Geometry: final body of the model. Coordinates: model frame, mm. Give positions to 0.01 mm unless a question says otherwise; leave off trailing zeros. Write each loop counter-clockwise with the first axis right and the second up, starting at its lowest first coordinate (ties: lowest second). Pieces come first, ordered by that corner, then holes. Notation, with made-up numbers: (26.5, 81.25) - (31.5, 81.25) arc R36 cw to (31.5, 116.25) - close; hole circle Ø6 at (76, 65). An arc over 180 degrees is marked (long way). Return JSON: item names as keys, results as strings.
from build123d import *

# Parameters (mm, degrees)
SKETCH1_R           = 2.5
BOSS_EXTRUDE1_DEPTH = 6.2
SKETCH2_R           = 2.5
CUT_EXTRUDE1_DEPTH  = 16.2


with BuildPart() as part:
    # Sketch1 → Boss-Extrude1 (new body)
    with BuildSketch(Plane.XY):
        with BuildLine():
            Line((0, 8), (33, 8))
            ThreePointArc((33, 8), (41, 0), (33, -8))
            Line((33, -8), (0, -8))
            ThreePointArc((0, -8), (-8, 0), (0, 8))
        make_face()
        with Locations(Location((0, 0, 0), (0, 0, 180))):
            Circle(SKETCH1_R, mode=Mode.SUBTRACT)
    extrude(amount=BOSS_EXTRUDE1_DEPTH)

    # Sketch2 → Cut-Extrude1 (cut)
    with BuildSketch(Plane.XY.offset(6.2)):
        with Locations((33, 0)):
            Circle(SKETCH2_R)
    extrude(amount=-CUT_EXTRUDE1_DEPTH, mode=Mode.SUBTRACT)


solid = part.part
Q1. Section query A-A, the plane y = 0. Return the cut outline in (x, z), plus the area to 3 significant figures.
Answer key:
{"outline": "(-8, 0) - (-2.5, 0) - (-2.5, 6.2) - (-8, 6.2) - close; (2.5, 0) - (30.5, 0) - (30.5, 6.2) - (2.5, 6.2) - close; (35.5, 0) - (41, 0) - (41, 6.2) - (35.5, 6.2) - close", "area": "242 mm^2"}
Q2. Section query C-C, the plane x = 38. Return the cut outline in (y, z) (3 decimals), plus the area to 3 significant figures.
Answer key:
{"outline": "(-6.245, 0) - (6.245, 0) - (6.245, 6.2) - (-6.245, 6.2) - close", "area": "77.4 mm^2"}
Q3. Material intervals for probe 1 along Y at (x, z) = (33, 2.75); probe 2 along X at (y, z) = (1, 4.25); probe 3 along X at (y, z) = (1.75, 4.25), sorted ascending. Write a range as [from, to].
Answer key:
{"probe 1": "y = [-8, -2.5], [2.5, 8]", "probe 2": "x = [-7.94, -2.29], [2.29, 30.71], [35.29, 40.94]", "probe 3": "x = [-7.81, -1.79], [1.79, 31.21], [34.79, 40.81]"}
Q4. Section query B-B, the plane z = 1.75. Return the cut outline in (x, y).
Answer key:
{"outline": "(0, -8) - (33, -8) arc R8 ccw to (33, 8) - (0, 8) arc R8 ccw to start; hole circle Ø5 at (0, 0); hole circle Ø5 at (33, 0)"}
Q5. Section query D-D, the plane y = -6.75. Return the cut outline in (x, z).
Answer key:
{"outline": "(-4.29, 0) - (37.29, 0) - (37.29, 6.2) - (-4.29, 6.2) - close"}
Q6. Mould query, pull axis Y, two halves, no side actions, for faces 1 (the cylindrical face through (35.31, -0.96, 3.14)), 2 (the flat face through (17, 0, 0)), 3 (the cylindrical face through (41, 0, 3)). Classes: pulls with the +Y half, pulls with the -Y half, needs draft (parallel to the pull), parting line crosses it, or undercut.
Answer key:
{"face 1": "undercut", "face 2": "needs draft", "face 3": "parting line crosses it"}
